Read the model definition and answer for the solid it produces. Units are mm, in the model's axes. A direction names the side the tool comes from. Give positions to 0.01 mm unless a question says otherwise; leave off trailing zeros. Write each loop counter-clockwise with the first axis right and the second up, starting at its lowest first coordinate (ties: lowest second). Pieces come first, ordered by that corner, then holes. Notation, with made-up numbers: M 28,-26.5 L 39,-26.5 A8 ccw 39,-19.5 Z; hole C 27.25,10 d3. An arc over 180 degrees is marked long. Use a Markdown table: item, result. Add a question column.
Item 1: Given P1, Ø5, axis at x = 18, y = 0, coming from the -Z side; P2, Ø1, axis at x = 17, y = -0.5, coming from the +Z side; P3, Ø4.5, axis at x = -18, y = 0, coming from the +Z side; P4, Ø3, axis at x = -9.5, z = 0, coming from the -Y side, each flat-ended and moving along its own axis, determine where each tip first touches the part or whether it passes through.
Item 2: A cutting plane is placed at D-D on z = 0. Determine the outline of the cut face in (x, y), then the cut area to 3 significant figures.
Item 3: A cutting plane is placed at A-A on z = 9.5. Determine the outline of the cut face in (x, y), then the cut area to 3 significant figures.
Item 4: A cutting plane is placed at B-B on x = 9.5. Determine the outline of the cut face in (y, z).
Item 5: For faces 4 (the flat face through (0, 0, -12.7)), 5 (the cylindrical face through (15.273, 0.358, -7.77)), 6 (the cylindrical face through (15.273, 0.358, 7.77)), determine the directions among +Z, -Z, +X, -X, +Y, -Y from which every point of the face is accessible in a straight line to the end or side of a thin tool.
Item 6: A cutting plane is placed at C-C on x = 0. Determine the outline of the cut face in (y, z).
Item 7: The mould has two halves that part along Y. Classify faces 1 (the flat face through (23.75, 0, 0)), 2 (the conical face through (-18.47, 0.06, -1.33)), 3 (the flat face through (0, 5, 0)): pulls with the +Y half, pulls with the -Y half, needs draft (parallel to the pull), parting line crosses it, or undercut.
Item 8: Consider probe 1 along X at (y, z) = (0, 5.25); probe 2 along Z at (x, y) = (0, -1.5); probe 3 along Y at (x, z) = (-18, -5). Determine where each line is inside the solid, lowest interval first. Write a range as [from, to].
from build123d import *

# Parameters (mm, degrees)
BOSS_EXTRUDE1_DEPTH                             = 5
CSK_FOR_M3_FLAT_HEAD_MACHINE_SCREW1_D           = 3.4
CSK_FOR_M3_FLAT_HEAD_MACHINE_SCREW1_CSINK_D     = 6.3
CSK_FOR_M3_FLAT_HEAD_MACHINE_SCREW1_CSINK_ANGLE = 90
F_5_5_5_5_DIAMETER_HOLE1_AT_2_COUNT             = 2
F_5_5_5_5_DIAMETER_HOLE1_AT_2_PITCH             = 36


with BuildPart() as part:
    # Sketch1 → Boss-Extrude1 (new body, symmetric)
    with BuildSketch(Plane(origin=(0, 0, 0), x_dir=(1, 0, 0), z_dir=(0, 1, 0))):
        Polygon((-23.75, 12.7), (-15.25, 12.7), (15.25, 12.7), (23.75, 12.7), (23.75, -12.7), (15.25, -12.7), (-15.25, -12.7), (-23.75, -12.7), align=None)
    extrude(amount=BOSS_EXTRUDE1_DEPTH, both=True)

    # CSK for M3 Flat Head Machine Screw1 (through all)
    with Locations(Plane(origin=(0, -5, 0), x_dir=(-1, 0, 0), z_dir=(0, -1, 0))):
        with Locations((-9.5, 0), (0, 9.5), (9.5, 0), (0, -9.5)):
            CounterSinkHole(CSK_FOR_M3_FLAT_HEAD_MACHINE_SCREW1_D / 2, CSK_FOR_M3_FLAT_HEAD_MACHINE_SCREW1_CSINK_D / 2, counter_sink_angle=CSK_FOR_M3_FLAT_HEAD_MACHINE_SCREW1_CSINK_ANGLE)

    # Sketch10 → Ø5.5 (5.5) Diameter Hole1 (revolve, cut)
    with BuildSketch(Plane(origin=(-18, 0, 12.7), x_dir=(0, -1, 0), z_dir=(1, 0, 0))):
        Polygon((0, 0), (0, 11.652366702), (2.75, 10), (2.75, 0), align=None)
    f_5_5_5_5_diameter_hole1 = revolve(axis=Axis((-18, 0, 19.05), (0, 0, -1)), mode=Mode.SUBTRACT)

    # Ø5.5 (5.5) Diameter Hole1 at 2: Ø5.5 (5.5) Diameter Hole1 ×2
    with Locations(*[(i * F_5_5_5_5_DIAMETER_HOLE1_AT_2_PITCH, 0, 0) for i in range(1, F_5_5_5_5_DIAMETER_HOLE1_AT_2_COUNT)]):
        add(f_5_5_5_5_diameter_hole1, mode=Mode.SUBTRACT)

    # Mirror1: Ø5.5 (5.5) Diameter Hole1 across plane
    add(f_5_5_5_5_diameter_hole1.mirror(Plane.XY), mode=Mode.SUBTRACT)

    # Mirror1 copy 1 sketch → Mirror1 copy 1 (revolve, cut)
    with BuildSketch(Plane(origin=(18, 0, -12.7), x_dir=(0, -1, 0), z_dir=(1, 0, 0))):
        Polygon((0, 0), (0, -11.652366702), (2.75, -10), (2.75, 0), align=None)
    revolve(axis=Axis((18, 0, -19.05), (0, 0, -1)), mode=Mode.SUBTRACT)


solid = part.part
Filled in:
| question | item | result |
|---|---|---|
| 1 | P1 | z = -2.55 |
| 1 | P2 | z = 2.02 |
| 1 | P3 | z = 2.4 |
| 1 | P4 | through |
| 2 | outline | M -23.75,-5 L -12.65,-5 L -11.2,-3.55 L -11.2,5 L -23.75,5 Z; M -7.8,-3.55 L -6.35,-5 L 6.35,-5 L 7.8,-3.55 L 7.8,5 L -7.8,5 Z; M 11.2,-3.55 L 12.65,-5 L 23.75,-5 L 23.75,5 L 11.2,5 Z |
| 2 | area | 403 mm² |
| 3 | outline | M -23.75,-5 L -3.15,-5 L -1.7,-3.55 L -1.7,5 L -23.75,5 Z; M 1.7,-3.55 L 3.15,-5 L 23.75,-5 L 23.75,5 L 1.7,5 Z; hole C -18,0 d5.5; hole C 18,0 d5.5 |
| 3 | area | 391 mm² |
| 4 | outline | M -5,-12.7 L 5,-12.7 L 5,-1.7 L -3.55,-1.7 L -5,-3.15 Z; M -5,3.15 L -3.55,1.7 L 5,1.7 L 5,12.7 L -5,12.7 Z |
| 5 | face 4 | -Z, +X, -X, +Y, -Y |
| 5 | face 5 | -Z |
| 5 | face 6 | +Z |
| 6 | outline | M -5,-12.7 L 5,-12.7 L 5,-11.2 L -3.55,-11.2 L -5,-12.65 Z; M -5,-6.35 L -3.55,-7.8 L 5,-7.8 L 5,7.8 L -3.55,7.8 L -5,6.35 Z; M -5,12.65 L -3.55,11.2 L 5,11.2 L 5,12.7 L -5,12.7 Z |
| 7 | face 1 | needs draft |
| 7 | face 2 | undercut |
| 7 | face 3 | pulls with the +Y half |
| 8 | probe 1 | [-23.75, -20.75], [-15.25, 15.25], [20.75, 23.75] |
| 8 | probe 2 | [-12.7, -11.2], [-7.8, 7.8], [11.2, 12.7] |
| 8 | probe 3 | [-5, -2.75], [2.75, 5] |
